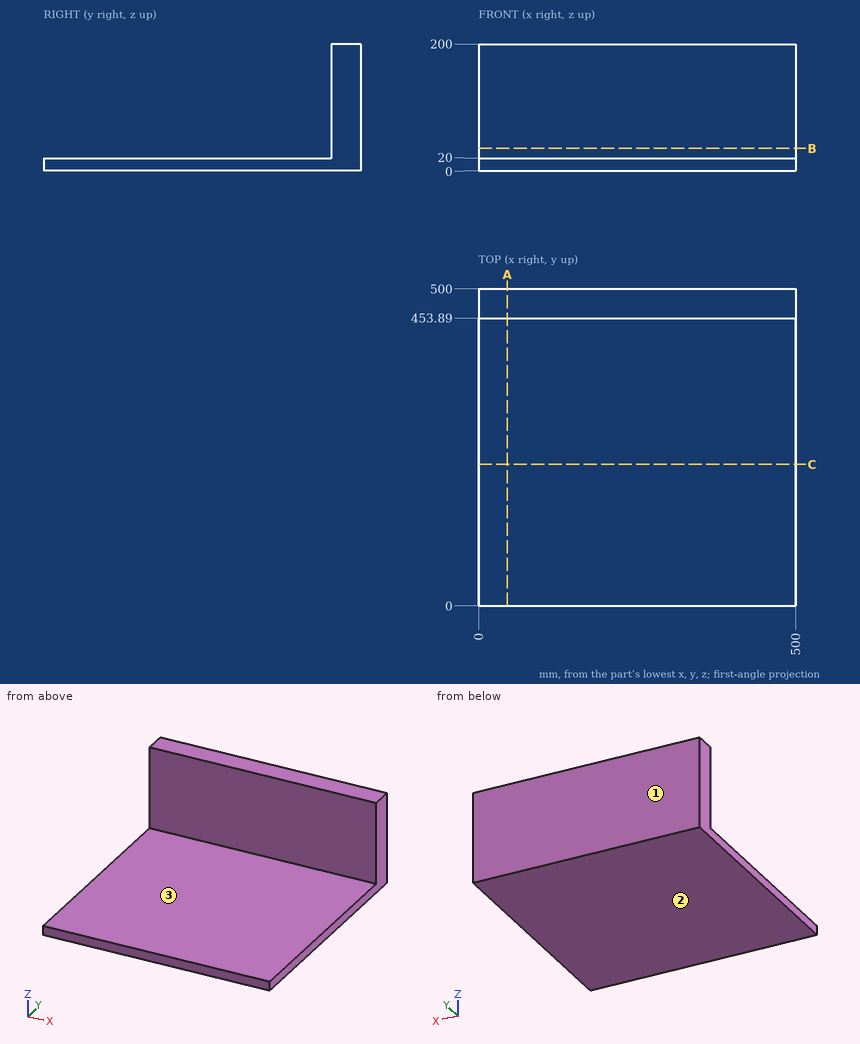
Verification items for this drawing (mm, ordinates from the low corner). Give positions to 0.01 mm unless a question says otherwise; leave off trailing zeros. Loops run counter-clockwise (first coordinate to the right, second up) from the corner with the lowest first, then second, coordinate; pieces in that order, holes last. Notation, with made-up numbers: M 54.5,-38.75 L 60.5,-38.75 A16 cw 60.5,-30.75 Z; hole C -0.5,65 d7. An arc over 180 degrees is marked long. Answer in a Markdown table with one row per item.
1) Depth check by flat-ended pin: pin 1 (2 mm diameter, centred on x = 344.5, z = 95.5, fed in from -Y); pin 2 (12 mm diameter, centred on x = 123.5, y = 195.5, fed in from +Z). Enter the tip coordinate at first touch or a pass-through.
Solutions:
| item | result |
|---|---|
| pin 1 | stops at y = 453.89 |
| pin 2 | stops at z = 20 |
2) Thickness scan on line 1 (Z direction, x = 216.5, y = 58); line 2 (Y direction, x = 103, z = 42). Record the ranges inside material, lowest first.
Solutions:
| item | result |
|---|---|
| line 1 | z = 0 to 20 |
| line 2 | y = 453.89 to 500 |
3) Mould release check, pull along Z, two halves, no side actions. Record for the marked faces 1, 2 and 3: released by +Z, released by -Z, zero draft, split by the parting line, or undercut.
Solutions:
| item | result |
|---|---|
| face 1 | zero draft |
| face 2 | released by -Z |
| face 3 | released by +Z |
4) Cross-section at A-A (x = 45.5). Enter the section's corners in (y, z).
Solutions:
| item | result |
|---|---|
| outline | M 0,0 L 500,0 L 500,200 L 453.89,200 L 453.89,20 L 0,20 Z |
5) Cross-section at C-C (y = 223). Enter the section's corners in (x, z), plus the area to 3 significant figures.
Solutions:
| item | result |
|---|---|
| outline | M 0,0 L 500,0 L 500,20 L 0,20 Z |
| area | 10,000 mm^2 |
6) Cross-section at B-B (z = 35.5). Enter the section's corners in (x, y), plus the area to 3 significant figures.
Solutions:
| item | result |
|---|---|
| outline | M 0,453.89 L 500,453.89 L 500,500 L 0,500 Z |
| area | 23,100 mm^2 |
